```python
from build123d import *

# Parameters (mm, degrees)
SKETCH1_W           = 35.8267
SKETCH1_H           = 54.2417
BOSS_EXTRUDE1_DEPTH = 6.35
SKETCH2_W           = 35.8267
SKETCH2_H           = 127
BOSS_EXTRUDE2_DEPTH = 6.35
BOSS_EXTRUDE3_DEPTH = 5.08
FILLET1_R           = 3.81
BOSS_EXTRUDE4_DEPTH = 6.35
SKETCH7_R           = 1.4986
CUT_EXTRUDE2_DEPTH  = 6.35


with BuildPart() as part:
    # Sketch1 → Boss-Extrude1 (new body)
    with BuildSketch(Plane.XY):
        Rectangle(SKETCH1_W, SKETCH1_H)
    extrude(amount=BOSS_EXTRUDE1_DEPTH)

    # Sketch2 → Boss-Extrude2 (add)
    with BuildSketch(Plane(origin=(0, 27.12085, 0), x_dir=(1, 0, 0), z_dir=(0, 1, 0))):
        with Locations((0, -63.5)):
            Rectangle(SKETCH2_W, SKETCH2_H)
    extrude(amount=-BOSS_EXTRUDE2_DEPTH)

    # Sketch4 → Boss-Extrude3 (add)
    with BuildSketch(Plane(origin=(17.91335, 0, 0), x_dir=(0, 0, -1), z_dir=(1, 0, 0))):
        Polygon((-6.35, 0), (-94.906446238, 20.77085), (-6.35, 20.77085), align=None)
    boss_extrude3 = extrude(amount=-BOSS_EXTRUDE3_DEPTH)

    # Mirror1: Boss-Extrude3 across plane
    add(boss_extrude3.mirror(Plane(origin=(0, 0, 0), x_dir=(0, 0, 1), z_dir=(1, 0, 0))))

    # Fillet1
    fillet1_edges = [part.edges().sort_by_distance(p)[0] for p in [
        (-17.91335, 23.94585, 127),
        (17.91335, 23.94585, 127),
        (15.37335, 0, 6.35),
        (15.37335, 20.77085, 94.906446238),
        (-15.37335, 0, 6.35),
        (-15.37335, 20.77085, 94.906446238),
        (17.91335, -27.12085, 3.175),
        (-17.91335, -27.12085, 3.175),
    ]]
    fillet(fillet1_edges, radius=FILLET1_R)

    # Sketch6 → Boss-Extrude4 (add)
    with BuildSketch(Plane(origin=(0, 27.12085, 0), x_dir=(1, 0, 0), z_dir=(0, 1, 0))):
        with BuildLine():
            Line((-66.04, -79.50835), (66.04, -79.50835))
            ThreePointArc((66.04, -79.50835), (68.734076836, -78.392426836), (69.85, -75.69835))
            Line((69.85, -75.69835), (69.85, -47.49165))
            ThreePointArc((69.85, -47.49165), (68.734076836, -44.797573164), (66.04, -43.68165))
            Line((66.04, -43.68165), (-66.04, -43.68165))
            ThreePointArc((-66.04, -43.68165), (-68.734076836, -44.797573164), (-69.85, -47.49165))
            Line((-69.85, -47.49165), (-69.85, -75.69835))
            ThreePointArc((-69.85, -75.69835), (-68.734076836, -78.392426836), (-66.04, -79.50835))
        make_face()
    extrude(amount=-BOSS_EXTRUDE4_DEPTH)

    # Sketch7 → Cut-Extrude2 (cut)
    with BuildSketch(Plane(origin=(0, 27.12085, 0), x_dir=(1, 0, 0), z_dir=(0, 1, 0))):
        with Locations((0, -21.840825)):
            Circle(SKETCH7_R)
        with Locations((39.754175, -61.595)):
            Circle(SKETCH7_R)
        with Locations((0, -101.349175)):
            Circle(SKETCH7_R)
        with Locations((-39.754175, -61.595)):
            Circle(SKETCH7_R)
    extrude(amount=-CUT_EXTRUDE2_DEPTH, mode=Mode.SUBTRACT)


solid = part.part
```
Build history of the part. All positions in model axes, mm. A direction names the side the tool comes from. Coordinates: 2 decimals unless noted, no trailing zeros. Order: outer loops, then holes, each group sorted by start corner. A loop starts at its lowest first (then second) coordinate and runs counter-clockwise, first axis right, second up.
Item 1: Saw through at C-C on x = -49.5. List the corners of the cut face in (y, z), then the cut area to 4 significant figures.
Filled in:
outline: (20.77, 43.68) - (27.12, 43.68) - (27.12, 79.51) - (20.77, 79.51) - close
area: 227.5 mm2
Item 2: Drop flat-ended pins along their axis: pin 1 Ø18 at (x, z) = (-55, 55.5) entering from -Y; pin 2 Ø10 at (y, z) = (20, 110.5) entering from +X; pin 3 Ø7 at (x, y) = (-54, 25) entering from +Z. Give the stop position or say it passes through.
Filled in:
pin 1: stops at y = 20.77
pin 2: stops at x = 17.91
pin 3: stops at z = 79.51
Item 3: Tool access for faces 4 (the flat face through (-42, 24, 79.508)), 5 (the flat face through (44, 20.771, 61)), 6 (the flat face through (12.833, 14, 30)), 7 (the flat face through (42, 24, 79.508)): list every direction of +Z, -Z, +X, -X, +Y, -Y with a clear straight run to the whole face (end or side of a thin tool).
Filled in:
face 4: +Z, -X, +Y, -Y
face 5: +Z, -Z, +X, -Y
face 6: +Z, -Y
face 7: +Z, +X, +Y, -Y
Item 4: Mould opens along Z. For faces 1 (the cylindrical face through (68.764, 23.99, 44.827)), 2 (the cylindrical face through (-0.325, 23.99, 102.812)), 3 (the flat face through (69.85, 24, 62)) say: released by +Z, released by -Z, zero draft, split by the parting line, or undercut.
Filled in:
face 1: released by -Z
face 2: undercut
face 3: zero draft
Item 5: Saw through at B-B on y = -5. List the corners of the cut face in (x, z).
Filled in:
outline: (-17.91, 0) - (17.91, 0) - (17.91, 6.35) - (-17.91, 6.35) - close
Item 6: Drill centre lines: L1, parallel to Z at x = 0, y = 22; L2, parallel to X at y = 11.5, z = 10.5; L3, parallel to Z at x = -5.5, y = 3. Where is each one in solid material? Low to high.
Filled in:
L1: z = 0 to 20.34, 23.34 to 99.85, 102.85 to 127
L2: x = -17.91 to -12.83, 12.83 to 17.91
L3: z = 0 to 6.35
Item 7: Saw through at A-A on z = 38. List the corners of the cut face in (x, y), then the cut area to 3 significant figures.
Filled in:
outline: (-17.91, 7.42) - (-12.83, 7.42) - (-12.83, 20.77) - (12.83, 20.77) - (12.83, 7.42) - (17.91, 7.42) - (17.91, 27.12) - (-17.91, 27.12) - close
area: 363 mm2
